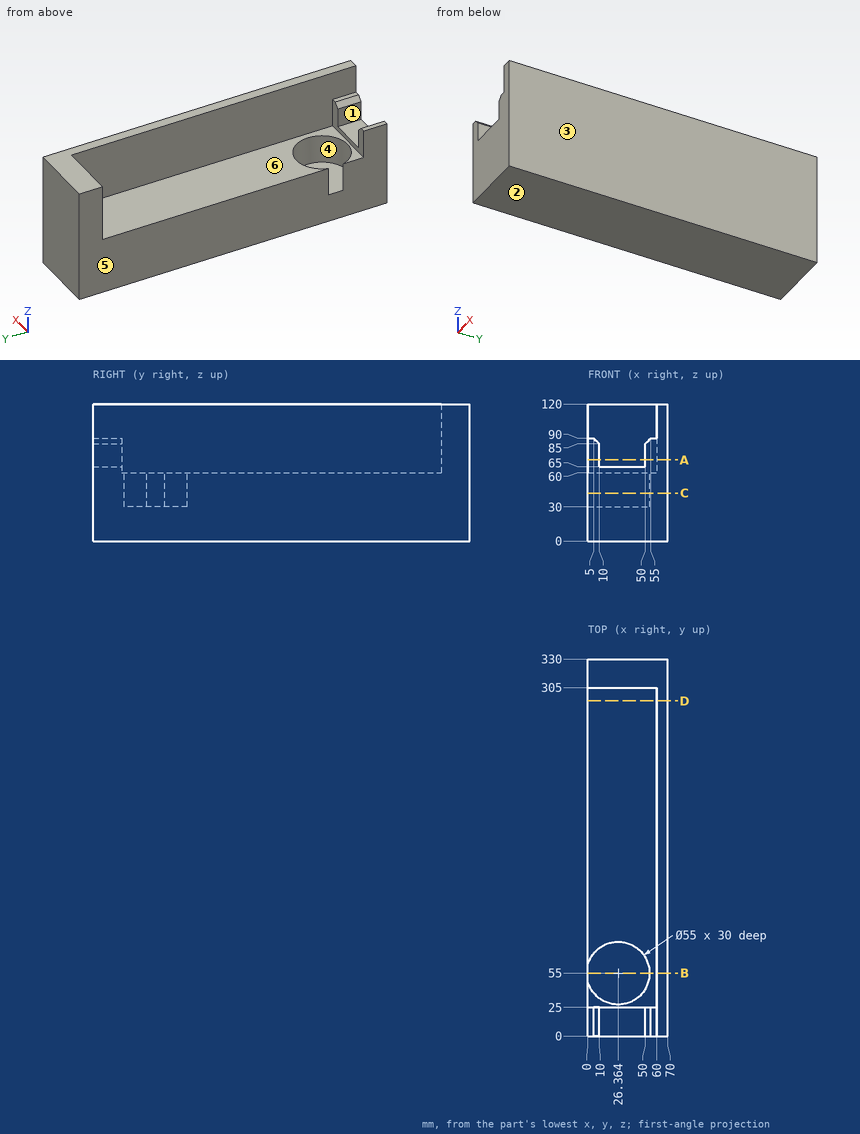
Answer from the drawing. Dimensions are ordinates in mm from the lowest x, y and z of the part. A direction names the side the tool comes from. Give positions to 0.01 mm unless a question says otherwise; leave off trailing zeros. Order: outer loops, then holes, each group sorted by start corner. A loop starts at its lowest first (then second) coordinate and runs counter-clockwise, first axis right, second up. Notation, with made-up numbers: (4.25, 63) -> (30.25, 63) arc R20 ccw to (30.25, 83) -> close; hole circle Ø4 at (24, 25). An arc over 180 degrees is marked (long way). One line per item, written item: value.
Item 1: Find section B-B, the plane y = 55. Give the vertices of the cut face in (x, z).
Answer sheet:
outline: (0, 0) -> (70, 0) -> (70, 120) -> (60, 120) -> (60, 60) -> (53.86, 60) -> (53.86, 30) -> (0, 30) -> close
Item 2: Determine the mould class of the marked faces 1, 2 and 3 for opening direction X: released by +X, released by -X, zero draft, split by the parting line, or undercut.
Answer sheet:
face 1: undercut
face 2: zero draft
face 3: released by +X
Item 3: A tool of negligible diameter and unlimited length cuts with its end or side. For the marked faces 4, 5 and 6, from which of +Z, -Z, +X, -X, +Y, -Y can it reach the whole face along a straight path? Write none if from no direction.
Answer sheet:
face 4: +Z
face 5: +Z, -Z, -X, +Y, -Y
face 6: +Z, -X
Item 4: Straight lines are drawn through the part: probe 1 along Y at (x, z) = (26, 44); probe 2 along Y at (x, z) = (59, 80); probe 3 along Z at (x, y) = (46.5, 163). For each, find the intervals that lie inside material, in ascending order.
Answer sheet:
probe 1: 0 to 27.5, 82.5 to 330
probe 2: 0 to 25, 305 to 330
probe 3: 0 to 60
Item 5: Find section A-A, the plane z = 71. Give the vertices of the cut face in (x, y).
Answer sheet:
outline: (0, 0) -> (10, 0) -> (10, 25) -> (0, 25) -> close; (0, 305) -> (60, 305) -> (60, 25) -> (50, 25) -> (50, 0) -> (70, 0) -> (70, 330) -> (0, 330) -> close
Item 6: Flat-ended cylindrical pins translate along their axes: P1, Ø5, axis at x = 20, y = 204.5, coming from the +Z side; P2, Ø2, axis at x = 41.5, y = 217, coming from the -Z side; P3, Ø16, axis at x = 20, y = 48.5, coming from the +Z side; P4, Ø20, axis at x = 35, y = 13, coming from the +Z side. Find the tip coordinate at first contact, or state that the pin passes through.
Answer sheet:
P1: z = 60
P2: z = 0
P3: z = 30
P4: z = 65
Item 7: Find section C-C, the plane z = 42. Give the vertices of the cut face in (x, y), plus the area to 3 significant figures.
Answer sheet:
outline: (0, 0) -> (70, 0) -> (70, 330) -> (0, 330) -> (0, 62.82) arc R27.5 cw (long way) to (0, 47.18) -> close
area: 20,700 mm²
Item 8: Find section D-D, the plane y = 293.5. Give the vertices of the cut face in (x, z), plus the area to 3 significant figures.
Answer sheet:
outline: (0, 0) -> (70, 0) -> (70, 120) -> (60, 120) -> (60, 60) -> (0, 60) -> close
area: 4,800 mm²
